```python
from build123d import *

# Parameters (mm, degrees)
F0_R     = 25.25
F0_R_2   = 12
F0_R_3   = 9.8
F1_DEPTH = 10
F0_R_4   = 32
F2_DEPTH = 3.25
F3_R     = 2


# Not quite as in the source:
# - a feature names something its author has since deleted; it is built from what else it names


with BuildPart() as f1:
    # F0 (on Top) → F1 (new body)
    with BuildSketch(Plane.XY):
        Circle(F0_R)
        Circle(F0_R_2, mode=Mode.SUBTRACT)
        Circle(F0_R_2)
        Circle(F0_R_3, mode=Mode.SUBTRACT)
    extrude(amount=F1_DEPTH)

    # F0 (on Top) → F2 (join)
    with BuildSketch(Plane.XY):
        Circle(F0_R_4)
        Circle(F0_R, mode=Mode.SUBTRACT)
    extrude(amount=F2_DEPTH)

    # F3
    f3_edges = [f1.edges().sort_by_distance(p)[0] for p in [
        (-25.25, 0, 10),
    ]]
    fillet(f3_edges, radius=F3_R)


solid = f1.part
```
Verification items for the finished model (mm, model axes). Give positions to 0.01 mm unless a question says otherwise; leave off trailing zeros. Write each loop counter-clockwise with the first axis right and the second up, starting at its lowest first coordinate (ties: lowest second). Pieces come first, ordered by that corner, then holes. Notation, with made-up numbers: (12.25, -12.75) - (32.25, -12.75) arc R29 ccw to (32.25, 25.25) - close; hole circle Ø3 at (76.5, 27.25). An arc over 180 degrees is marked (long way). Put each result on its own line as item: value.
Q1. Scan lines: probe 1 along Y at (x, z) = (0, 2); probe 2 along Y at (x, z) = (0, 6); probe 3 along Z at (x, y) = (-27, -9.5). Record each from-to range of solid material in increasing order. Write a range as from..to.
Result:
probe 1: -32..-9.8, 9.8..32
probe 2: -25.25..-9.8, 9.8..25.25
probe 3: 0..3.25
Q2. Section check C-C on z = 2. Record the cut outline in (x, y), and give its area (3 significant figures).
Result:
outline: circle Ø64 at (0, 0); hole circle Ø19.6 at (0, 0)
area: 2,920 mm2
Q3. Section check D-D on x = 28.5. Record the cut outline in (y, z).
Result:
outline: (-14.55, 0) - (14.55, 0) - (14.55, 3.25) - (-14.55, 3.25) - close
Q4. Depth check by flat-ended pin: P1, Ø4, axis at y = 9, z = 5.5, coming from the +X side; P2, Ø3, axis at y = -24.5, z = 8.5, coming from the +X side; P3, Ø6, axis at y = 25, z = 5, coming from the +X side. Enter the tip coordinate at first touch or a pass-through.
Result:
P1: x = 24.26
P2: x = 10.34
P3: x = 22.69
Q5. Mould release check, pull along X, two halves, no side actions. Record for faces 1 (the face through (-2.124, -9.567, 4.93)), 2 (the face through (24, 10, 3.25)), 3 (the face through (-5.47, -24.65, 5.59)): released by +X, released by -X, zero draft, split by the parting line, or undercut.
Result:
face 1: undercut
face 2: zero draft
face 3: split by the parting line
Q6. Section check A-A on y = 0. Record the cut outline in (x, z).
Result:
outline: (-32, 0) - (-9.8, 0) - (-9.8, 10) - (-23.25, 10) arc R2 ccw to (-25.25, 8) - (-25.25, 3.25) - (-32, 3.25) - close; (9.8, 0) - (32, 0) - (32, 3.25) - (25.25, 3.25) - (25.25, 8) arc R2 ccw to (23.25, 10) - (9.8, 10) - close
